Work out the finished part from the listing and answer in its coordinate system (mm). A direction names the side the tool comes from. Give positions to 0.01 mm unless a question says otherwise; leave off trailing zeros. Loops run counter-clockwise (first coordinate to the right, second up) from the corner with the lowest first, then second, coordinate; pieces in that order, holes last. Notation, with made-up numbers: M 68.25,-27.75 L 94.25,-27.75 A25 cw 94.25,1.25 Z; hole C 68.5,-14 d8. An arc over 180 degrees is marked long. Use a Markdown table: item, result.
```python
from build123d import *

# Parameters (mm, degrees)
AUFSATZ_LINEAR_AUSTRAGEN1_DEPTH = 10
DURCHGANGSLOCH_F_R_M31_D        = 3.4
FORMSCHR_GE1_ANGLE              = 45


with BuildPart() as part:
    # Skizze1 → Aufsatz-Linear austragen1 (new body)
    with BuildSketch(Plane(origin=(0, 0, 0), x_dir=(1, 0, 0), z_dir=(0, 1, 0))):
        Polygon((0, 0), (-4.55, 0), (-4.55, -1), (-6.55, -1), (-6.55, 1), (-2.95, 1), (-2.95, 2), (0, 2), align=None)
    extrude(amount=AUFSATZ_LINEAR_AUSTRAGEN1_DEPTH)

    # Spiegeln1: part across plane


with BuildPart() as part_1:
    add(part.part)
    add(part.part.mirror(Plane(origin=(0, 10, -2), x_dir=(0, 0, 1), z_dir=(-1, 0, 0))))

    # Durchgangsloch für M31 (through all)
    with Locations(Plane.XY):
        with Locations((0, 5)):
            Hole(DURCHGANGSLOCH_F_R_M31_D / 2)

    # Formschräge1
    formschr_ge1_faces = [part_1.faces().sort_by_distance(p)[0] for p in [
        (4.55, 5, 0.5),
        (-4.55, 5, 0.5),
    ]]
    draft(formschr_ge1_faces, Plane(origin=(0, 10, 0), x_dir=(1, 0, 0), z_dir=(0, 0, 1)), FORMSCHR_GE1_ANGLE)


solid = part_1.part
```
(1) A cutting plane is placed at A-A (z = 0.25). Write down the section's boundary in (x, y), and give its area (3 significant figures).
Entries:
| item | result |
|---|---|
| outline | M -6.55,0 L -4.8,0 L -4.8,10 L -6.55,10 Z; M 4.8,0 L 6.55,0 L 6.55,10 L 4.8,10 Z |
| area | 35.0 mm² |
(2) The mould has two halves that part along X. Classify faces 1 (the flat face through (-5, 5, -1)), 2 (the cylindrical face through (0.37, 3.34, -1.01)), 3 (the flat face through (6.55, 5, 0)): released by +X, released by -X, zero draft, split by the parting line, or undercut.
Entries:
| item | result |
|---|---|
| face 1 | zero draft |
| face 2 | undercut |
| face 3 | released by +X |
(3) Consider probe 1 along Y at (x, z) = (0, -1.3); probe 2 along Z at (x, y) = (-2.5, 3.5); probe 3 along X at (y, z) = (5.25, -1.1). Determine where each line is inside the solid, lowest interval first. Write a range as [from, to].
Entries:
| item | result |
|---|---|
| probe 1 | y = [0, 3.3], [6.7, 10] |
| probe 2 | z = [-2, 0] |
| probe 3 | x = [-2.95, -1.68], [1.68, 2.95] |
(4) Which of the six approach directions +Z, -Z, +X, -X, +Y, -Y give full straight-line access (tool end or side, diameter ignored) to faces 4 (the flat face through (2.95, 4.9, -1.5)), 5 (the flat face through (0, 10, -1)), 6 (the flat face through (-2, 5, 0)), 7 (the flat face through (2, 5, -2)), 8 (the flat face through (-2.95, 4.9, -1.5))?
Entries:
| item | result |
|---|---|
| face 4 | -Z, +X, +Y, -Y |
| face 5 | +Z, -Z, +X, -X, +Y |
| face 6 | +Z, +Y, -Y |
| face 7 | -Z, +X, -X, +Y, -Y |
| face 8 | -Z, -X, +Y, -Y |
(5) A cutting plane is placed at D-D (y = 1.75). Write down the section's boundary in (x, z).
Entries:
| item | result |
|---|---|
| outline | M -6.55,-1 L -2.95,-1 L -2.95,-2 L 2.95,-2 L 2.95,-1 L 6.55,-1 L 6.55,1 L 5.55,1 L 4.55,0 L -4.55,0 L -5.55,1 L -6.55,1 Z |
(6) A cutting plane is placed at C-C (x = 0). Write down the section's boundary in (y, z), and give its area (3 significant figures).
Entries:
| item | result |
|---|---|
| outline | M 0,-2 L 3.3,-2 L 3.3,0 L 0,0 Z; M 6.7,-2 L 10,-2 L 10,0 L 6.7,0 Z |
| area | 13.2 mm² |
(7) Given P1, Ø4.5, axis at x = 0, y = 5, coming from the +Z side; P2, Ø0.5, axis at y = 5, z = -1.5, coming from the -X side; P3, Ø0.5, axis at y = 3.5, z = -1.5, coming from the +X side, each flat-ended and moving along its own axis, determine where each tip first touches the part or whether it passes through.
Entries:
| item | result |
|---|---|
| P1 | stops at z = 0 |
| P2 | stops at x = -2.95 |
| P3 | stops at x = 2.95 |
(8) A cutting plane is placed at B-B (y = 3.5). Write down the section's boundary in (x, z), and give its area (3 significant figures).
Entries:
| item | result |
|---|---|
| outline | M -6.55,-1 L -2.95,-1 L -2.95,-2 L -0.8,-2 L -0.8,0 L -4.55,0 L -5.55,1 L -6.55,1 Z; M 0.8,-2 L 2.95,-2 L 2.95,-1 L 6.55,-1 L 6.55,1 L 5.55,1 L 4.55,0 L 0.8,0 Z |
| area | 18.8 mm² |
